```python
from build123d import *

# Parameters (mm, degrees)
BLANKSKE_W              = 80
BLANKSKE_H              = 7.5
BLANK_DEPTH             = 20
TOOTHCUTSIM_DEPTH       = 83.802475808
TEETHCUTS_COUNT         = 18
TEETHCUTS_PITCH         = 4.712388975
SKETCH1_W               = 20
SKETCH1_H               = 11.625
BOSS_EXTRUDE2_DEPTH     = 7.5
SKETCH3_W               = 20
SKETCH3_H               = 15
BOSS_EXTRUDE3_DEPTH     = 7.5
SKETCH4_W               = 7.5
SKETCH4_H               = 15
BOSS_EXTRUDE4_DEPTH     = 15
SKETCH8_W               = 7.5
SKETCH8_H               = 7.5
CUT_EXTRUDE1_DEPTH      = 15
CUT_EXTRUDE2_DEPTH      = 15
SKETCH10_W              = 7.5
SKETCH10_H              = 7.5
BOSS_EXTRUDE5_DEPTH     = 7.5
SKETCH11_W              = 7.5
SKETCH11_H              = 15
BOSS_EXTRUDE7_DEPTH     = 60
CUT_EXTRUDE4_DEPTH      = 116.829144109
CUT_EXTRUDE4_DEPTH_BACK = 116.829144109
SKETCH12_W              = 95
SKETCH12_H              = 10
SKETCH14_W              = 95
SKETCH14_H              = 2.5
CUT_EXTRUDE5_DEPTH      = 100
SKETCH15_W              = 67.5
SKETCH15_H              = 7.5
CUT_EXTRUDE6_DEPTH      = 122.963109177
BOSS_EXTRUDE8_DEPTH     = 7.5
BOSS_EXTRUDE9_DEPTH     = 1


with BuildPart() as part:
    # BlankSke → Blank (new body)
    with BuildSketch(Plane.XY):
        with Locations((40, 3.75)):
            Rectangle(BLANKSKE_W, BLANKSKE_H)
    extrude(amount=-BLANK_DEPTH)

    # TooCutSkeSim → ToothCutSim (cut, through all)
    with BuildSketch(Plane.XY):
        Polygon((0.654653055, 4.125), (-0.654653055, 4.125), (-1.892297439, 7.5254), (1.892297439, 7.5254), align=None)
    toothcutsim = extrude(amount=-TOOTHCUTSIM_DEPTH, mode=Mode.SUBTRACT)

    # TeethCuts: ToothCutSim ×18
    with Locations(*[(i * TEETHCUTS_PITCH, 0, 0) for i in range(1, TEETHCUTS_COUNT)]):
        add(toothcutsim, mode=Mode.SUBTRACT)

    # Sketch1 → Boss-Extrude2 (add)
    with BuildSketch(Plane(origin=(80, 0, 0), x_dir=(0, 0, -1), z_dir=(1, 0, 0))):
        with Locations((10, -1.6875)):
            Rectangle(SKETCH1_W, SKETCH1_H)
    extrude(amount=BOSS_EXTRUDE2_DEPTH)

    # Sketch3 → Boss-Extrude3 (add)
    with BuildSketch(Plane.ZY):
        with Locations((-10, 7.5)):
            Rectangle(SKETCH3_W, SKETCH3_H)
    extrude(amount=BOSS_EXTRUDE3_DEPTH)

    # Sketch4 → Boss-Extrude4 (add)
    with BuildSketch(Plane.XY):
        with Locations((-3.75, 7.5)):
            Rectangle(SKETCH4_W, SKETCH4_H)
    extrude(amount=BOSS_EXTRUDE4_DEPTH)

    # Sketch8 → Cut-Extrude1 (cut)
    with BuildSketch(Plane(origin=(0, 0, 0), x_dir=(0, 0, -1), z_dir=(1, 0, 0))):
        with Locations((-3.75, 3.75)):
            Rectangle(SKETCH8_W, SKETCH8_H)
    extrude(amount=-CUT_EXTRUDE1_DEPTH, mode=Mode.SUBTRACT)

    # Sketch9 → Cut-Extrude2 (cut)
    with BuildSketch(Plane.ZY.offset(7.5)):
        Polygon((7.5, 15), (15, 7.5), (15, 15), align=None)
    extrude(amount=-CUT_EXTRUDE2_DEPTH, mode=Mode.SUBTRACT)

    # Sketch10 → Boss-Extrude5 (add)
    with BuildSketch(Plane.XZ):
        with Locations((-3.75, 11.25)):
            Rectangle(SKETCH10_W, SKETCH10_H)
    extrude(amount=BOSS_EXTRUDE5_DEPTH)

    # Sketch11 → Boss-Extrude7 (add)
    with BuildSketch(Plane.XY.offset(15)):
        with Locations((-3.75, 0)):
            Rectangle(SKETCH11_W, SKETCH11_H)
    extrude(amount=BOSS_EXTRUDE7_DEPTH)

    # Sketch12 → Cut-Extrude4 (cut, two sides: drawn at the far end of the back side and taken through both)
    with BuildSketch(Plane(origin=(0, 4.125, 0), x_dir=(1, 0, 0), z_dir=(0, 1, 0)).offset(-CUT_EXTRUDE4_DEPTH_BACK)):
        with Locations((40, 15)):
            Rectangle(SKETCH12_W, SKETCH12_H)
    extrude(amount=CUT_EXTRUDE4_DEPTH + CUT_EXTRUDE4_DEPTH_BACK, mode=Mode.SUBTRACT)

    # Sketch14 → Cut-Extrude5 (cut)
    with BuildSketch(Plane(origin=(0, 15, 0), x_dir=(1, 0, 0), z_dir=(0, 1, 0))):
        with Locations((40, 8.75)):
            Rectangle(SKETCH14_W, SKETCH14_H)
    extrude(amount=-CUT_EXTRUDE5_DEPTH, mode=Mode.SUBTRACT)

    # Sketch15 → Cut-Extrude6 (cut, through all)
    with BuildSketch(Plane.ZY.offset(7.5)):
        with Locations((41.25, -3.75)):
            Rectangle(SKETCH15_W, SKETCH15_H)
    extrude(amount=-CUT_EXTRUDE6_DEPTH, mode=Mode.SUBTRACT)

    # Sketch16 → Boss-Extrude8 (add)
    with BuildSketch(Plane.ZY.offset(7.5)):
        with BuildLine():
            Line((7.5, 7.5), (7.5, 15))
            ThreePointArc((7.5, 15), (12.803300859, 12.803300859), (15, 7.5))
            Line((15, 7.5), (7.5, 7.5))
        make_face()
    extrude(amount=-BOSS_EXTRUDE8_DEPTH)

    # Sketch19 → Boss-Extrude9 (add)
    with BuildSketch(Plane.XY):
        Polygon((-7.5, 0), (-7.5, 7.5), (0, 7.5), (0, 4.125), (87.5, 4.125), (87.5, -7.5), (80, -7.5), (80, 0), align=None)
    extrude(amount=BOSS_EXTRUDE9_DEPTH)


solid = part.part
```
Source: CAD feature listing. Evaluate the final solid. Frame: model axes, mm. A direction names the side the tool comes from. Round coordinates to 2 decimals unless told otherwise and drop trailing zeros. Order: outer loops, then holes, each group sorted by start corner. A loop starts at its lowest first (then second) coordinate and runs counter-clockwise, first axis right, second up. Notation, with made-up numbers: (89, 74.5) -> (121, 74.5) arc R24 ccw to (121, 110.5) -> close; hole circle Ø5 at (56, 53). An arc over 180 degrees is marked (long way). Use CSV: the item, a comma, the result in double quotes.
(1) Section B-B on z = 64. Return the cut outline in (x, y).
Report:
outline,"(-7.5, 0) -> (0, 0) -> (0, 7.5) -> (-7.5, 7.5) -> close"
(2) Section A-A on y = 1.25. Return the cut outline in (x, z).
Report:
outline,"(-7.5, -7.5) -> (87.5, -7.5) -> (87.5, 1) -> (-7.5, 1) -> close; (-7.5, 7.5) -> (0, 7.5) -> (0, 75) -> (-7.5, 75) -> close"
(3) Pull-direction query (X, two-part tool) for faces 4 (the face through (78, 5, 0)), 5 (the face through (1.28, 5.84, -3.7)), 6 (the face through (87.5, -2, -3)); classes: +X half, -X half, draft (parallel to the pull), parting line (faces both ways), or undercut.
Report:
face 4,"draft"
face 5,"undercut"
face 6,"+X half"
(4) First-contact query: pin 1 Ø3.5 at (x, y) = (45, 5.5) entering from +Z; pin 2 Ø5 at (x, y) = (45, -3) entering from +Z; pin 3 Ø10 at (y, z) = (6, 32) entering from +X; pin 4 Ø0.5 at (x, z) = (63.5, -4.5) entering from +Y. Flat tips, straight axial feed; report the tip coordinate or a pass-through.
Report:
pin 1,"z = 1"
pin 2,"through"
pin 3,"x = 0"
pin 4,"y = 7.5"
(5) Ray query, L1, parallel to Z at x = -2.5, y = 2; L2, parallel to Z at x = 27, y = 4.5; L3, parallel to Z at x = 60, y = 2.25. Return the intervals inside material, ascending.
Report:
L1,"-7.5 to 1, 7.5 to 75"
L2,"-7.5 to 0"
L3,"-7.5 to 1"
(6) Section C-C on y = 11.5. Return the cut outline in (x, z), and give its area (3 significant figures).
Report:
outline,"(-7.5, -7.5) -> (0, -7.5) -> (0, 13.84) -> (-7.5, 13.84) -> close"
area,"160 mm^2"
(7) Access query for faces 1 (the face through (12, 5, 0)), 2 (the face through (20.13, 5.84, -3.7)), 3 (the face through (41, 2, 1)). Directions: +Z, -Z, +X, -X, +Y, -Y. A direction counts if a zero-diameter tool reaches every point of the face in a straight line with its end or side. Return the directions, or none.
Report:
face 1,"+Z, +X, +Y"
face 2,"+Z, -Z, +Y"
face 3,"+X, -X, -Y"
